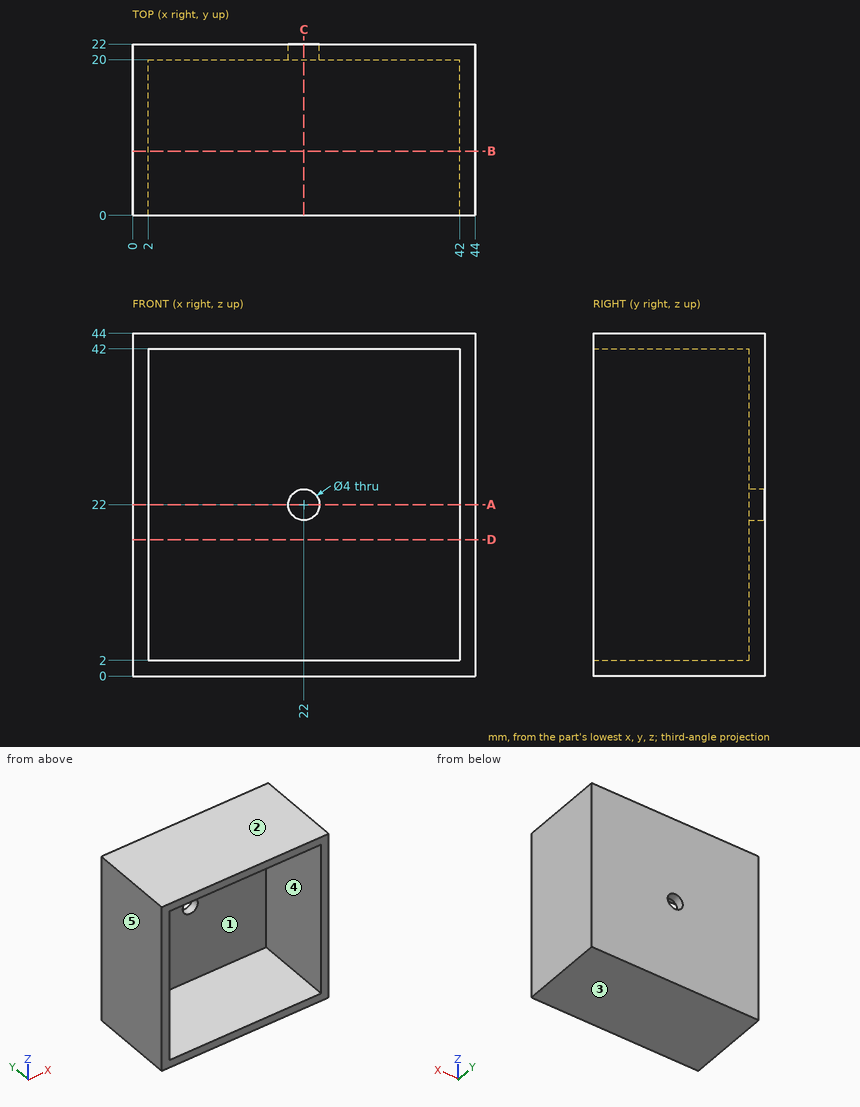
Job drawing, mm, ordinate dimensions from the low corner. One solid piece. A direction names the side the tool comes from. Round coordinates to 2 decimals unless told otherwise and drop trailing zeros. Loops run counter-clockwise (first coordinate to the right, second up) from the corner with the lowest first, then second, coordinate; pieces in that order, holes last.
Item 1: 3-axis set-ups, long thin cutter, end or side, ignore diameter. For the marked faces 1 and 2: which of +Z, -Z, +X, -X, +Y, -Y reach the whole face in a straight line?
Item 2: Cut at A-A, the plane z = 22. Give the cut face in (x, y), then the cut area to 3 significant figures.
Item 3: Cut at B-B, the plane y = 8.25. Give the cut face in (x, z).
Item 4: Cut at C-C, the plane x = 22. Give the cut face in (y, z), then the cut area to 3 significant figures.
Item 5: Mould opens along X. For the marked faces 3, 4 and 5 say: +X half, -X half, draft (parallel to the pull), parting line (faces both ways), or undercut.
Item 6: Drill centre lines: line 1 (Z direction, x = 23, y = 17.25); line 2 (X direction, y = 21.6, z = 22). Where is each one in solid material? Low to high.
Item 7: Drop flat-ended pins along their axis: P1, Ø6, axis at y = 8, z = 26, coming from the -X side; P2, Ø8, axis at x = 13, z = 31.5, coming from the -Y side. Give the stop position or say it passes through.
Item 8: Cut at D-D, the plane z = 17.5. Give the cut face in (x, y).
A:
1. face 1: -Y
1. face 2: +Z, +X, -X, +Y, -Y
2. outline: (0, 0) - (2, 0) - (2, 20) - (20, 20) - (20, 22) - (0, 22) - close; (24, 20) - (42, 20) - (42, 0) - (44, 0) - (44, 22) - (24, 22) - close
2. area: 160 mm2
3. outline: (0, 0) - (44, 0) - (44, 44) - (0, 44) - close; hole (2, 2) - (42, 2) - (42, 42) - (2, 42) - close
4. outline: (0, 0) - (22, 0) - (22, 20) - (20, 20) - (20, 2) - (0, 2) - close; (0, 42) - (20, 42) - (20, 24) - (22, 24) - (22, 44) - (0, 44) - close
4. area: 160 mm2
5. face 3: draft
5. face 4: undercut
5. face 5: -X half
6. line 1: z = 0 to 2, 42 to 44
6. line 2: x = 0 to 20, 24 to 44
7. P1: stops at x = 0
7. P2: stops at y = 20
8. outline: (0, 0) - (2, 0) - (2, 20) - (42, 20) - (42, 0) - (44, 0) - (44, 22) - (0, 22) - close
